Check sheet for the modelled part. Datum: model origin and axes. Units: mm. A direction names the side the tool comes from. Coordinates: 2 decimals unless noted, no trailing zeros. Loops run counter-clockwise (first coordinate to the right, second up) from the corner with the lowest first, then second, coordinate; pieces in that order, holes last. Notation, with made-up numbers: (54, 34) -> (80, 34) arc R20 cw to (80, 64) -> close; hole circle Ø11 at (71.5, 1.5). An arc over 180 degrees is marked (long way). Use CSV: the item, a comma, the result in double quotes. Start each with the question number.
1. Sectioned sample at A-A, the plane y = -19.15. Record the cut outline in (x, z), and give its area (3 significant figures).
2. Sectioned sample at B-B, the plane x = 5.5. Record the cut outline in (y, z).
3. Set-up check for faces 5 (the face through (46.5, 9, -2)), 6 (the face through (-20.5, 0, -3)): record each of +Z, -Z, +X, -X, +Y, -Y from which the full face is reachable in a straight line by a thin tool's end or side.
4. Thickness scan on L1, parallel to Y at x = -24, z = -2.3; L2, parallel to Y at x = -5, z = -0.5; L3, parallel to X at y = 0.5, z = -2.5. Record the ranges inside material, lowest first.
5. Gauge pin test, flat ends, axial feed: pin 1 (6 mm diameter, centred on y = 16, z = 3.5, fed in from -X); pin 2 (7.5 mm diameter, centred on x = 1.5, z = 10, fed in from -Y); pin 3 (4 mm diameter, centred on x = 8, y = 17, fed in from +Z); pin 4 (4 mm diameter, centred on x = -24, y = -5, fed in from -Z). Record the tip position at first contact, or that the pin passes through.
6. Sectioned sample at D-D, the plane x = 32.5. Record the cut outline in (y, z).
7. Release check for a two-part mould opening along Z. For faces 1 (the face through (39.03, 26.57, 9.73)), 2 (the face through (8, 23.15, 7)), 3 (the face through (8, 11, 0)), 4 (the face through (-20.92, 26.57, 9.82)) record: pulls with the +Z half, pulls with the -Z half, needs draft (parallel to the pull), parting line crosses it, or undercut.
8. Sectioned sample at C-C, the plane y = 5. Record the cut outline in (x, z), and give its area (3 significant figures).
```python
from build123d import *

# Parameters (mm, degrees)
SKETCH1_W           = 75
SKETCH1_H           = 46.3
SKETCH1_R           = 1.5
SKETCH1_W_2         = 41
SKETCH1_H_2         = 20
BASE_FLANGE2_DEPTH  = 6
EDGE_FLANGE1_DEPTH  = 75
CUT_EXTRUDE1_REACH  = 74.112
SKETCH15_R          = 1.6
CUT_EXTRUDE2_REACH  = 61.131
SKETCH16_R          = 1.6
SKETCH17_W          = 75
SKETCH17_H          = 21
BOSS_EXTRUDE1_DEPTH = 6.7366
CUT_EXTRUDE3_REACH  = 74.112
SKETCH18_R          = 1.6


# Sheet-metal steps are written as plain solids
with BuildPart() as part:
    # Sketch1 → Base-Flange2 (new body)
    with BuildSketch(Plane.XY):
        with Locations((9, 0)):
            Rectangle(SKETCH1_W, SKETCH1_H)
        with Locations((-24, 5)):
            Circle(SKETCH1_R, mode=Mode.SUBTRACT)
        with Locations(Location((24, 5, 0), (0, 0, 180))):
            Circle(SKETCH1_R, mode=Mode.SUBTRACT)
        with Locations((24, -5)):
            Circle(SKETCH1_R, mode=Mode.SUBTRACT)
        with Locations(Location((-24, -5, 0), (0, 0, 180))):
            Circle(SKETCH1_R, mode=Mode.SUBTRACT)
        Rectangle(SKETCH1_W_2, SKETCH1_H_2, mode=Mode.SUBTRACT)
    extrude(amount=-BASE_FLANGE2_DEPTH)

    # Edge-Flange1 section (across the edge) → Edge-Flange1 (add)
    with BuildSketch(Plane(origin=(46.5, 23.8866, 0), x_dir=(0, -1, 0), z_dir=(-1, 0, 0))):
        with BuildLine():
            Line((-6, 0.7366), (-6, 15))
            Line((-6, 15), (0, 15))
            Line((0, 15), (0, 0.7366))
            ThreePointArc((0, 0.7366), (0.215745145, 0.215745145), (0.7366, 0))
            Line((0.7366, 0), (0.7366, -6))
            ThreePointArc((0.7366, -6), (-4.026895542, -4.026895542), (-6, 0.7366))
        make_face()
    extrude(amount=EDGE_FLANGE1_DEPTH)

    # Sketch15 → Cut-Extrude1 (cut, up to next)
    with BuildSketch(Plane(origin=(0, 29.8866, 0), x_dir=(1, 0, 0), z_dir=(0, 1, 0)), mode=Mode.PRIVATE) as cut_extrude1_sk1:
        with Locations(Location((-22, -11, 0), (0, 0, 270))):
            Circle(SKETCH15_R)
    cut_extrude1_tool1 = extrude(cut_extrude1_sk1.sketch, amount=-CUT_EXTRUDE1_REACH, mode=Mode.PRIVATE) & part.part
    # Sketch15 → Cut-Extrude1 (cut, up to next)
    with BuildSketch(Plane(origin=(0, 29.8866, 0), x_dir=(1, 0, 0), z_dir=(0, 1, 0)), mode=Mode.PRIVATE) as cut_extrude1_sk2:
        with Locations(Location((40, -11, 0), (0, 0, 90))):
            Circle(SKETCH15_R)
    cut_extrude1_tool2 = extrude(cut_extrude1_sk2.sketch, amount=-CUT_EXTRUDE1_REACH, mode=Mode.PRIVATE) & part.part
    add(cut_extrude1_tool1.solids().sort_by_distance((-22, 29.8866, 11))[0], mode=Mode.SUBTRACT)
    add(cut_extrude1_tool2.solids().sort_by_distance((40, 29.8866, 11))[0], mode=Mode.SUBTRACT)

    # Sketch16 → Cut-Extrude2 (cut, up to next)
    with BuildSketch(Plane(origin=(0, 0, -6), x_dir=(-1, 0, 0), z_dir=(0, 0, -1)), mode=Mode.PRIVATE) as cut_extrude2_sk1:
        with Locations((-42.5, -19.15)):
            Circle(SKETCH16_R)
    cut_extrude2_tool1 = extrude(cut_extrude2_sk1.sketch, amount=-CUT_EXTRUDE2_REACH, mode=Mode.PRIVATE) & part.part
    # Sketch16 → Cut-Extrude2 (cut, up to next)
    with BuildSketch(Plane(origin=(0, 0, -6), x_dir=(-1, 0, 0), z_dir=(0, 0, -1)), mode=Mode.PRIVATE) as cut_extrude2_sk2:
        with Locations((-11.5, -19.15)):
            Circle(SKETCH16_R)
    cut_extrude2_tool2 = extrude(cut_extrude2_sk2.sketch, amount=-CUT_EXTRUDE2_REACH, mode=Mode.PRIVATE) & part.part
    add(cut_extrude2_tool1.solids().sort_by_distance((42.5, -19.15, -6))[0], mode=Mode.SUBTRACT)
    add(cut_extrude2_tool2.solids().sort_by_distance((11.5, -19.15, -6))[0], mode=Mode.SUBTRACT)

    # Sketch17 → Boss-Extrude1 (add)
    with BuildSketch(Plane(origin=(0, 29.8866, 0), x_dir=(1, 0, 0), z_dir=(0, 1, 0))):
        with Locations((9, -4.5)):
            Rectangle(SKETCH17_W, SKETCH17_H)
    extrude(amount=-BOSS_EXTRUDE1_DEPTH)

    # Sketch18 → Cut-Extrude3 (cut, up to next)
    with BuildSketch(Plane(origin=(0, 29.8866, 0), x_dir=(1, 0, 0), z_dir=(0, 1, 0)), mode=Mode.PRIVATE) as cut_extrude3_sk1:
        with Locations(Location((-22, -11, 0), (0, 0, 270))):
            Circle(SKETCH18_R)
    cut_extrude3_tool1 = extrude(cut_extrude3_sk1.sketch, amount=-CUT_EXTRUDE3_REACH, mode=Mode.PRIVATE) & part.part
    # Sketch18 → Cut-Extrude3 (cut, up to next)
    with BuildSketch(Plane(origin=(0, 29.8866, 0), x_dir=(1, 0, 0), z_dir=(0, 1, 0)), mode=Mode.PRIVATE) as cut_extrude3_sk2:
        with Locations(Location((40, -11, 0), (0, 0, 270))):
            Circle(SKETCH18_R)
    cut_extrude3_tool2 = extrude(cut_extrude3_sk2.sketch, amount=-CUT_EXTRUDE3_REACH, mode=Mode.PRIVATE) & part.part
    add(cut_extrude3_tool1.solids().sort_by_distance((-22, 29.8866, 11))[0], mode=Mode.SUBTRACT)
    add(cut_extrude3_tool2.solids().sort_by_distance((40, 29.8866, 11))[0], mode=Mode.SUBTRACT)


solid = part.part
```
Completed:
1,outline,"(-28.5, -6) -> (9.9, -6) -> (9.9, 0) -> (-28.5, 0) -> close; (13.1, -6) -> (40.9, -6) -> (40.9, 0) -> (13.1, 0) -> close; (44.1, -6) -> (46.5, -6) -> (46.5, 0) -> (44.1, 0) -> close"
1,area,"412 mm²"
2,outline,"(-23.15, -6) -> (-10, -6) -> (-10, 0) -> (-23.15, 0) -> close; (10, -6) -> (29.89, -6) -> (29.89, 15) -> (23.15, 15) -> (23.15, 0) -> (10, 0) -> close"
3,face 5,"+Z, -Z, +X, +Y, -Y"
3,face 6,"+Z, -Z"
4,L1,"-23.15 to -6.5, -3.5 to 3.5, 6.5 to 29.89"
4,L2,"-23.15 to -10, 10 to 29.89"
4,L3,"-28.5 to -20.5, 20.5 to 46.5"
5,pin 1,"through"
5,pin 2,"y = 23.15"
5,pin 3,"z = 0"
5,pin 4,"z = -6"
6,outline,"(-23.15, -6) -> (29.89, -6) -> (29.89, 15) -> (23.15, 15) -> (23.15, 0) -> (-23.15, 0) -> close"
7,face 1,"undercut"
7,face 2,"needs draft"
7,face 3,"pulls with the +Z half"
7,face 4,"undercut"
8,outline,"(-28.5, -6) -> (-25.5, -6) -> (-25.5, 0) -> (-28.5, 0) -> close; (-22.5, -6) -> (-20.5, -6) -> (-20.5, 0) -> (-22.5, 0) -> close; (20.5, -6) -> (22.5, -6) -> (22.5, 0) -> (20.5, 0) -> close; (25.5, -6) -> (46.5, -6) -> (46.5, 0) -> (25.5, 0) -> close"
8,area,"168 mm²"
